Can you work these out from the drawing? Everything is in mm from the part's minimum corner. A direction names the side the tool comes from. Coordinates: 2 decimals unless noted, no trailing zeros. Order: outer loops, then holes, each group sorted by start corner. A loop starts at its lowest first (then second) coordinate and runs counter-clockwise, first axis right, second up. Notation, with made-up numbers: (0, -36) - (11, -36) arc R11 ccw to (11, -15) - close; hole circle Ø3 at (52.5, -1). An arc over 180 degrees is marked (long way). Answer as CSV lines item,"result". Start each with the question number.
Item 1: Imagine slicing it at C-C on z = 27.5. List the corners of the cut face in (x, y) for me, and give its area (3 significant figures).
Item 2: I'm going to push flat-ended pins straight in: pin 1 (1.8 mm diameter, centred on y = 9.5, z = 66.5, fed in from +X) (1 decimal); pin 2 (5 mm diameter, centred on y = 3.5, z = 13, fed in from -X); pin 3 (9.5 mm diameter, centred on x = 17, z = 63, fed in from -Y); pin 4 (1.8 mm diameter, centred on y = 10.5, z = 64, fed in from -X). Where does each tip first touch, or does it pass through?
Item 3: Imagine slicing it at A-A on z = 59. List the corners of the cut face in (x, y) for me (1 decimal), and give its area (3 significant figures).
Item 4: Imagine slicing it at B-B on x = 46.5. List the corners of the cut face in (y, z) for me, and give its area (3 significant figures).
Item 5: We'd pull the mould along X, two halves only. Please class the marked faces 1 and 2: pulls with the +X half, pulls with the -X half, needs draft (parallel to the pull), parting line crosses it, or undercut.
Item 6: On a 3-axis mill with a long thin cutter (end or side, diameter ignored), from which of +Z, -Z, +X, -X, +Y, -Y can I reach the whole of each face in a straight line? I mean the marked faces 3, 4 and 5. Say none if no direction works.
Item 7: I need wall thicknesses on line 1 (X direction, y = 6.25, z = 40.5) (1 decimal); line 2 (Z direction, x = 32.5, y = 9); line 3 (X direction, y = 8.5, z = 62.5) (1 decimal). Which ranges of each line are inside material? Lowest first, please.
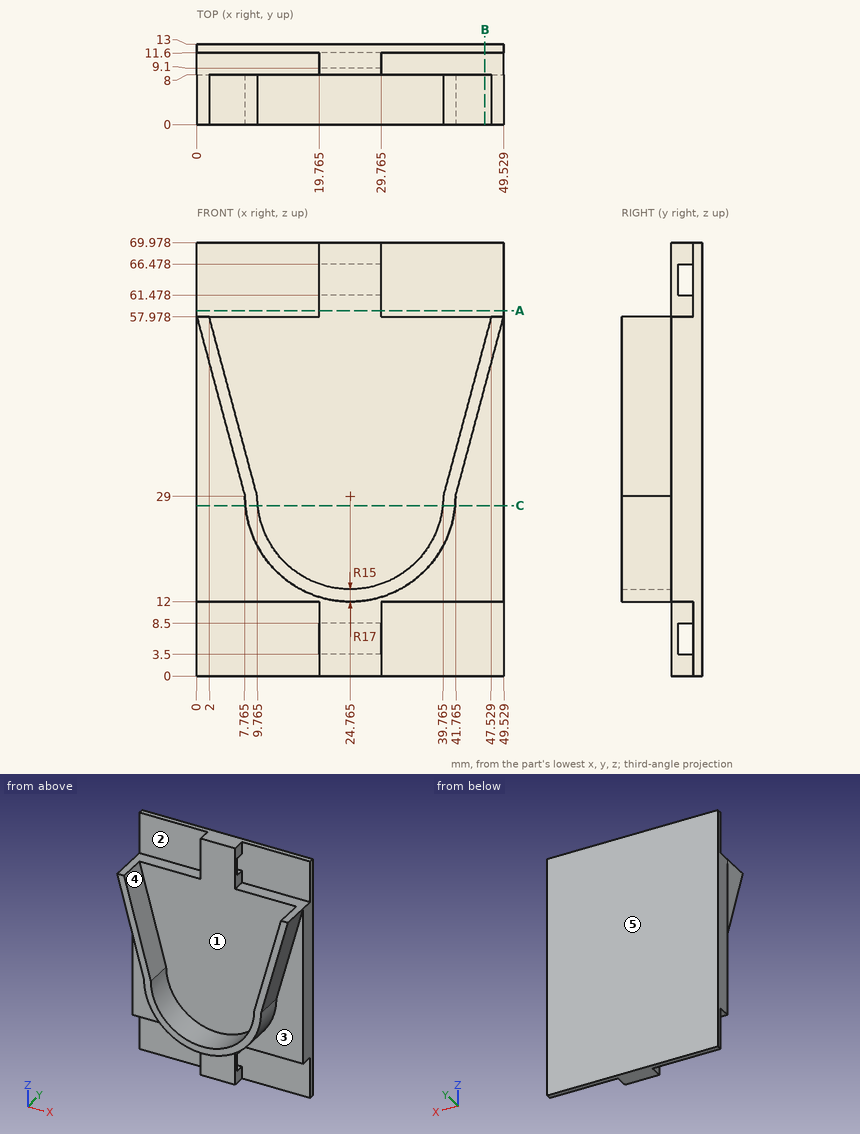
Responses:
1,outline,"(0, 8) - (7.83, 8) - (7.83, 0) - (9.84, 0) - (9.84, 8) - (39.69, 8) - (39.69, 0) - (41.7, 0) - (41.7, 8) - (49.53, 8) - (49.53, 13) - (0, 13) - close"
1,area,"280 mm^2"
2,pin 1,"stops at x = 29.8"
2,pin 2,"stops at x = 14.43"
2,pin 3,"stops at y = 8"
2,pin 4,"passes through"
3,outline,"(0, 11.6) - (19.8, 11.6) - (19.8, 8) - (29.8, 8) - (29.8, 11.6) - (49.5, 11.6) - (49.5, 13) - (0, 13) - close"
3,area,"105 mm^2"
4,outline,"(0, 46.67) - (8, 46.67) - (8, 12) - (11.6, 12) - (11.6, 0) - (13, 0) - (13, 69.98) - (11.6, 69.98) - (11.6, 57.98) - (8, 57.98) - (8, 54.14) - (0, 54.14) - close"
4,area,"323 mm^2"
5,face 1,"undercut"
5,face 2,"needs draft"
6,face 3,"-Z, -Y"
6,face 4,"+Z, -Y"
6,face 5,"+Z, -Z, +X, -X, +Y"
7,line 1,"x = 4.7 to 6.7, 42.8 to 44.8"
7,line 2,"z = 12 to 57.98"
7,line 3,"x = 19.8 to 29.8"
